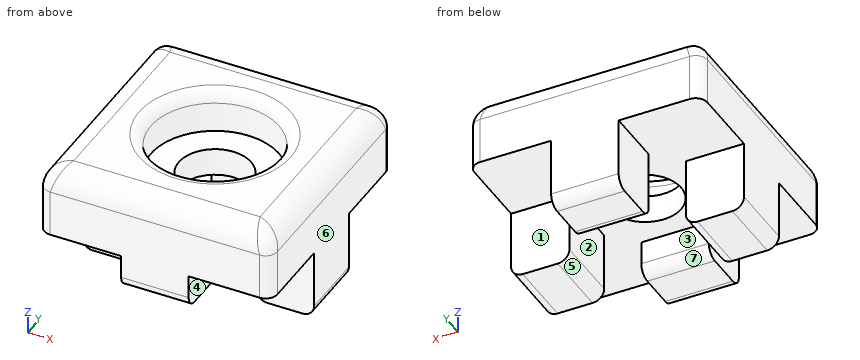
from build123d import *

# Parameters (mm, degrees)
SKETCH_W        = 20
SKETCH_H        = 20
PAD_DEPTH       = 6
SKETCH001_R     = 5.5
POCKET_DEPTH    = 3.6
SKETCH002_R     = 3.1
POCKET001_DEPTH = 5
SKETCH003_W     = 5.8
SKETCH003_H     = 5
PAD001_DEPTH    = 6
SKETCH004_W     = 5
SKETCH004_H     = 5.8
PAD002_DEPTH    = 6
SKETCH005_W     = 5.8
SKETCH005_H     = 5
PAD003_DEPTH    = 6
SKETCH006_W     = 5
SKETCH006_H     = 5.8
PAD004_DEPTH    = 6
SKETCH007_W     = 7.342915
SKETCH007_H     = 6.002037
POCKET002_DEPTH = 3
FILLET_R        = 1
FILLET001_R     = 1
FILLET002_R     = 2
FILLET003_R     = 1


with BuildPart() as part:
    # Sketch → Pad (new body)
    with BuildSketch(Plane.XY):
        with Locations((10, 10)):
            Rectangle(SKETCH_W, SKETCH_H)
    extrude(amount=PAD_DEPTH)

    # Sketch001 (on Face6 of Pad) → Pocket (cut)
    with BuildSketch(Plane.XY.offset(6)):
        with Locations((10, 10)):
            Circle(SKETCH001_R)
    extrude(amount=-POCKET_DEPTH, mode=Mode.SUBTRACT)

    # Sketch002 (on Face8 of Pocket) → Pocket001 (cut)
    with BuildSketch(Plane.XY.offset(2.4)):
        with Locations((10, 10)):
            Circle(SKETCH002_R)
    extrude(amount=-POCKET001_DEPTH, mode=Mode.SUBTRACT)

    # Sketch003 (on Face4 of Pocket001) → Pad001 (join)
    with BuildSketch(Plane(origin=(0, 0, 0), x_dir=(1, 0, 0), z_dir=(0, 0, -1))):
        with Locations((10, -2.5)):
            Rectangle(SKETCH003_W, SKETCH003_H)
    extrude(amount=PAD001_DEPTH)

    # Sketch004 (on Face4 of Pad001) → Pad002 (join)
    with BuildSketch(Plane(origin=(0, 0, 0), x_dir=(1, 0, 0), z_dir=(0, 0, -1))):
        with Locations((17.5, -10)):
            Rectangle(SKETCH004_W, SKETCH004_H)
    extrude(amount=PAD002_DEPTH)

    # Sketch005 (on Face4 of Pad002) → Pad003 (join)
    with BuildSketch(Plane(origin=(0, 0, 0), x_dir=(1, 0, 0), z_dir=(0, 0, -1))):
        with Locations((10, -17.5)):
            Rectangle(SKETCH005_W, SKETCH005_H)
    extrude(amount=PAD003_DEPTH)

    # Sketch006 (on Face4 of Pad003) → Pad004 (join)
    with BuildSketch(Plane(origin=(0, 0, 0), x_dir=(1, 0, 0), z_dir=(0, 0, -1))):
        with Locations((2.5, -10)):
            Rectangle(SKETCH006_W, SKETCH006_H)
    extrude(amount=PAD004_DEPTH)

    # Sketch007 → Pocket002 (cut)
    with BuildSketch(Plane(origin=(0, 0, -6), x_dir=(1, 0, 0), z_dir=(0, 0, -1))):
        with Locations((10.087635, -2.302989)):
            Rectangle(SKETCH007_W, SKETCH007_H)
    extrude(amount=-POCKET002_DEPTH, mode=Mode.SUBTRACT)

    # Fillet
    fillet_edges = [part.edges().sort_by_distance(p)[0] for p in [
        (10, 0, -3),
        (10, 5, -3),
        (5, 10, -6),
        (0, 10, -6),
        (10, 15, -6),
        (10, 20, -6),
        (15, 10, -6),
        (20, 10, -6),
    ]]
    fillet(fillet_edges, radius=FILLET_R)

    # Fillet001
    fillet001_edges = [part.edges().sort_by_distance(p)[0] for p in [
        (0, 20, 3),
        (20, 20, 3),
        (20, 0, 3),
        (0, 0, 3),
    ]]
    fillet(fillet001_edges, radius=FILLET001_R)

    # Fillet002
    fillet002_edges = [part.edges().sort_by_distance(p)[0] for p in [
        (10, 20, 6),
        (19.707107, 19.707107, 6),
        (20, 10, 6),
        (19.707107, 0.292893, 6),
        (10, 0, 6),
        (0.292893, 0.292893, 6),
        (0, 10, 6),
        (0.292893, 19.707107, 6),
    ]]
    fillet(fillet002_edges, radius=FILLET002_R)

    # Fillet003
    fillet003_edges = [part.edges().sort_by_distance(p)[0] for p in [
        (4.5, 10, 6),
    ]]
    fillet(fillet003_edges, radius=FILLET003_R)


solid = part.part
For this review, take the finished solid that the model builds, in its own axes (mm). Face numbers are marked on the shaded views. A direction names the side the tool comes from. Give positions to 0.01 mm unless a question says otherwise; leave off trailing zeros. Loops run counter-clockwise (first coordinate to the right, second up) from the corner with the lowest first, then second, coordinate; pieces in that order, holes last.
Item 1: Take a section at B-B, the plane x = 10. State the section outline as (y, z) points, and give its area (3 significant figures).
Item 2: Draft analysis for pull direction X (two halves, no side actions). For the marked faces 5, 6 and 7, state which applies: +X half, -X half, draft (parallel to the pull), parting line (faces both ways), or undercut.
Item 3: Tool access review of the marked faces 1, 2, 3 and 4: name each direction out of +Z, -Z, +X, -X, +Y, -Y from which nothing blocks a thin tool from reaching the whole face with its end or side.
Item 4: Insertion check: pin 1 (0.9 mm diameter, centred on y = 3.5, z = -1, fed in from +X); pin 2 (0.9 mm diameter, centred on y = 1.5, z = -1.5, fed in from -X); pin 3 (4 mm diameter, centred on x = 17.5, z = -2.5, fed in from -Y). Each pin has a flat end and moves straight along its axis. Give the tip position at first contact, or say it passes through.
Item 5: Take a section at C-C, the plane y = 10. State the section outline as (x, z) points, and give its area (3 significant figures).
Item 6: Take a section at A-A, the plane z = -3.75. State the section outline as (x, y) points, and give its area (3 significant figures).
Item 7: For line 1 along Y through (x, z) = (10, 1.05); line 2 along X through (y, z) = (7.5, -2.5); line 3 along Z through (x, y) = (13, 3.5), list the stretches that pass through material, from the lowest coordinate up.
Calculated:
1. outline: (0, -2) arc R1 ccw to (1, -3) - (4, -3) arc R1 ccw to (5, -2) - (5, 0) - (6.9, 0) - (6.9, 2.4) - (4.5, 2.4) - (4.5, 5) arc R1 ccw to (3.5, 6) - (2, 6) arc R2 ccw to (0, 4) - close; (13.1, 0) - (15, 0) - (15, -5) arc R1 ccw to (16, -6) - (19, -6) arc R1 ccw to (20, -5) - (20, 4) arc R2 ccw to (18, 6) - (16.5, 6) arc R1 ccw to (15.5, 5) - (15.5, 2.4) - (13.1, 2.4) - close
1. area: 108 mm2
2. face 5: undercut
2. face 6: +X half
2. face 7: draft
3. face 1: -Z, +X, -X, +Y
3. face 2: -Z, +Y, -Y
3. face 3: -Z, +X, -X
3. face 4: -Z, +X, +Y, -Y
4. pin 1: stops at x = 12.9
4. pin 2: stops at x = 7.1
4. pin 3: stops at y = 7.1
5. outline: (0, -5) arc R1 ccw to (1, -6) - (4, -6) arc R1 ccw to (5, -5) - (5, 0) - (6.9, 0) - (6.9, 2.4) - (4.5, 2.4) - (4.5, 5) arc R1 ccw to (3.5, 6) - (2, 6) arc R2 ccw to (0, 4) - close; (13.1, 0) - (15, 0) - (15, -5) arc R1 ccw to (16, -6) - (19, -6) arc R1 ccw to (20, -5) - (20, 4) arc R2 ccw to (18, 6) - (16.5, 6) arc R1 ccw to (15.5, 5) - (15.5, 2.4) - (13.1, 2.4) - close
5. area: 123 mm2
6. outline: (0, 7.1) - (5, 7.1) - (5, 12.9) - (0, 12.9) - close; (7.1, 15) - (12.9, 15) - (12.9, 20) - (7.1, 20) - close; (15, 7.1) - (20, 7.1) - (20, 12.9) - (15, 12.9) - close
6. area: 87.0 mm2
7. line 1: y = 0 to 6.9, 13.1 to 20
7. line 2: x = 0 to 5, 15 to 20
7. line 3: z = 0 to 6
